CAD build for the part. Positions are in the model's coordinates, mm. A direction names the side the tool comes from. Give positions to 0.01 mm unless a question says otherwise; leave off trailing zeros. Write each loop counter-clockwise with the first axis right and the second up, starting at its lowest first coordinate (ties: lowest second). Pieces come first, ordered by that corner, then holes. Notation, with made-up numbers: (85.5, 51.5) - (140.5, 51.5) arc R12 cw to (140.5, 64.5) - close; hole circle Ø2 at (-10.5, 84). An arc over 180 degrees is marked (long way). Answer as a JSON object with one key per item and string values.
from build123d import *

# Parameters (mm, degrees)
CROQUIS1_W                  = 6
CROQUIS1_H                  = 8
SALIENTE_EXTRUIR1_DEPTH     = 5
REDONDEO4_R                 = 1.5
SKETCH6_R                   = 4
CUT_EXTRUDE1_DEPTH          = 10
TAP_DRILL_FOR_M3X0_5_TAP1_D = 2.5


with BuildPart() as part:
    # Croquis1 → Revolución1 (revolve)
    with BuildSketch(Plane(origin=(0, 0, 0), x_dir=(0, 0, -1), z_dir=(1, 0, 0)), mode=Mode.PRIVATE) as revoluci_n1_sk:
        with Locations((-3, 4)):
            Rectangle(CROQUIS1_W, CROQUIS1_H)
    revolve(revoluci_n1_sk.sketch.rotate(Axis((0, 0, 0), (0, 1, 0)), 180), axis=Axis((0, 0, 0), (0, 1, 0)))

    # Croquis2 → Saliente-Extruir1 (add)
    with BuildSketch(Plane(origin=(0, 8, 0), x_dir=(1, 0, 0), z_dir=(0, 1, 0))):
        Polygon((-9.95, 0), (-4.975, -8.616952768), (4.975, -8.616952768), (9.95, 0), (4.975, 8.616952768), (-4.975, 8.616952768), align=None)
    extrude(amount=SALIENTE_EXTRUIR1_DEPTH)

    # Redondeo4
    redondeo4_edges = [part.edges().sort_by_distance(p)[0] for p in [
        (0, 8, 6),
    ]]
    fillet(redondeo4_edges, radius=REDONDEO4_R)

    # Sketch6 → Cut-Extrude1 (cut)
    with BuildSketch(Plane.XZ):
        with Locations(Location((0, 0, 0), (0, 0, 270))):
            Circle(SKETCH6_R)
    extrude(amount=-CUT_EXTRUDE1_DEPTH, mode=Mode.SUBTRACT)

    # Tap Drill for M3x0.5 Tap1 (through all)
    with Locations(Plane(origin=(0, 3.25, 6), x_dir=(1, 0, 0), z_dir=(0, 0, 1))):
        with Locations((0, 0)):
            Hole(TAP_DRILL_FOR_M3X0_5_TAP1_D / 2)


solid = part.part
(1) Saw through at D-D, the plane y = 11.25. Give the cut face in (x, z) (3 decimals), and give its area (3 significant figures).
Answer key:
{"outline": "(-9.95, 0) - (-4.975, -8.617) - (4.975, -8.617) - (9.95, 0) - (4.975, 8.617) - (-4.975, 8.617) - close", "area": "257 mm²"}
(2) Probe L1, parallel to X at y = 3, z = 0; L2, parallel to Y at x = 0, z = 4.6; L3, parallel to Z at x = -2.5, y = 2.25. List the from-to ranges inside material, lowest first. Write a range as [from, to].
Answer key:
{"L1": "x = [-6, -4], [4, 6]", "L2": "y = [0, 2], [4.5, 13]", "L3": "z = [-5.45, -3.12], [3.12, 5.45]"}
(3) Flat gauge pins, fed straight in: P1, Ø2, axis at y = 5, z = -0.5, coming from the -X side; P2, Ø4, axis at x = 2.5, y = 3, coming from the -Z side; P3, Ø2, axis at x = -6, y = 1.5, coming from the -Z side. Where does each tip first touch, or does it go through?
Answer key:
{"P1": "stops at x = -6", "P2": "stops at z = -5.96", "P3": "stops at z = -3.32"}
(4) Saw through at A-A, the plane x = 0. Give the cut face in (y, z).
Answer key:
{"outline": "(0, -6) - (2, -6) - (2, -4) - (0, -4) - close; (0, 4) - (2, 4) - (2, 6) - (0, 6) - close; (4.5, -6) - (6.5, -6) arc R1.5 cw to (8, -7.5) - (8, -8.62) - (13, -8.62) - (13, 8.62) - (8, 8.62) - (8, 7.5) arc R1.5 cw to (6.5, 6) - (4.5, 6) - (4.5, 4) - (10, 4) - (10, -4) - (4.5, -4) - close"}
(5) Pull direction Z, two halves, no side cores. Call faces 1 (the face through (0, 10, 0)), 2 (the face through (3.92, 0, 1.42)), 3 (the face through (0, 10, 8.617)): pulls with the +Z half, pulls with the -Z half, needs draft (parallel to the pull), parting line crosses it, or undercut.
Answer key:
{"face 1": "undercut", "face 2": "needs draft", "face 3": "pulls with the +Z half"}
(6) Saw through at C-C, the plane y = 5.25. Give the cut face in (x, z).
Answer key:
{"outline": "circle Ø12 at (0, 0); hole circle Ø8 at (0, 0)"}
(7) 3-axis set-ups, long thin cutter, end or side, ignore diameter. For faces 4 (the face through (-1.532, 4.93, -3.695)), 5 (the face through (-7.428, 10.465, -4.369)): which of +Z, -Z, +X, -X, +Y, -Y reach the whole face in a straight line?
Answer key:
{"face 4": "-Y", "face 5": "-Z, -X, +Y, -Y"}
(8) Saw through at B-B, the plane y = 3.25. Give the cut face in (x, z), and give its area (3 significant figures).
Answer key:
{"outline": "(-1.25, -5.87) - (-1.25, -3.8) arc R4 cw to (-1.25, 3.8) - (-1.25, 5.87) arc R6 ccw to start; (1.25, -5.87) arc R6 ccw to (1.25, 5.87) - (1.25, 3.8) arc R4 cw to (1.25, -3.8) - close", "area": "52.7 mm²"}
